from build123d import *

# Parameters (mm, degrees)
BOSS_EXTRUDE1_DEPTH = 3
SKETCH2_R           = 13.5
BOSS_EXTRUDE2_DEPTH = 5
SKETCH3_R           = 7.5
CUT_EXTRUDE1_DEPTH  = 1
SKETCH4_R           = 4
CUT_EXTRUDE2_DEPTH  = 9


with BuildPart() as part:
    # Sketch1 → Boss-Extrude1 (new body)
    with BuildSketch(Plane.XY):
        Polygon((5.773502692, -10), (11.547005384, 0), (5.773502692, 10), (-5.773502692, 10), (-11.547005384, 0), (-5.773502692, -10), align=None)
    extrude(amount=BOSS_EXTRUDE1_DEPTH)

    # Sketch2 → Boss-Extrude2 (add)
    with BuildSketch(Plane.XY.offset(3)):
        Circle(SKETCH2_R)
    extrude(amount=BOSS_EXTRUDE2_DEPTH)

    # Sketch3 → Cut-Extrude1 (cut)
    with BuildSketch(Plane.XY.offset(8)):
        Circle(SKETCH3_R)
    extrude(amount=-CUT_EXTRUDE1_DEPTH, mode=Mode.SUBTRACT)

    # Sketch4 → Cut-Extrude2 (cut, through all)
    with BuildSketch(Plane(origin=(0, 0, 0), x_dir=(-1, 0, 0), z_dir=(0, 0, -1))):
        Circle(SKETCH4_R)
    extrude(amount=-CUT_EXTRUDE2_DEPTH, mode=Mode.SUBTRACT)


solid = part.part
Verification items for the finished model (mm, model axes). A direction names the side the tool comes from. Give positions to 0.01 mm unless a question says otherwise; leave off trailing zeros. Loops run counter-clockwise (first coordinate to the right, second up) from the corner with the lowest first, then second, coordinate; pieces in that order, holes last. Notation, with made-up numbers: (85, 86) - (107, 86) arc R10 cw to (107, 103) - close; hole circle Ø7 at (38.25, 25.5). An arc over 180 degrees is marked (long way). Write item = value, one per line. Start each with the question number.
Q1. Cross-section at C-C, the plane y = 1. Enter the section's corners in (x, z).
Q2. Depth check by flat-ended pin: P1, Ø3, axis at x = 10, z = 2.5, coming from the -Y side; P2, Ø3, axis at y = -4.5, z = 6.5, coming from the +X side; P3, Ø1.5, axis at x = 9.5, z = 5.5, coming from the +Y side. Enter the tip coordinate at first touch or a pass-through.
Q3. Cross-section at A-A, the plane x = 3.5. Enter the section's corners in (y, z).
Q4. Thickness scan on line 1 (Y direction, x = 0, z = 7.4); line 2 (Y direction, x = 0, z = 2); line 3 (Z direction, x = 1.5, y = 4). Record the ranges inside material, lowest first.
Q5. Mould release check, pull along Y, two halves, no side actions. Record for faces 1 (the face through (0.867, -3.905, 3.451)), 2 (the face through (-8.7, -4.93, 1.48)), 3 (the face through (0, 10, 1)): released by +Y, released by -Y, zero draft, split by the parting line, or undercut.
Q6. Tool access check on faces 4 (the face through (8.62, -5.07, 1.48)), 5 (the face through (-8.62, 5.07, 1.48)), 6 (the face through (9, 5, 3)), 7 (the face through (-7.493, 0.33, 7.507)), 8 (the face through (8.7, 4.93, 1.48)). Record the directions out of +Z, -Z, +X, -X, +Y, -Y that give a thin tool (end or side, any length) a straight path to the whole face; none if there is none.
Q7. Cross-section at D-D, the plane z = 3.75. Enter the section's corners in (x, y).
Q8. Cross-section at B-B, the plane z = 1.25. Enter the section's corners in (x, y), and give its area (3 significant figures).
Answer key:
q1.outline = (-13.46, 3) - (-10.97, 3) - (-10.97, 0) - (-3.87, 0) - (-3.87, 7) - (-7.43, 7) - (-7.43, 8) - (-13.46, 8) - close; (3.87, 0) - (10.97, 0) - (10.97, 3) - (13.46, 3) - (13.46, 8) - (7.43, 8) - (7.43, 7) - (3.87, 7) - close
q2.P1 = -10.42
q2.P2 = 13.16
q2.P3 = 10.28
q3.outline = (-13.04, 3) - (-10, 3) - (-10, 0) - (-1.94, 0) - (-1.94, 7) - (-6.63, 7) - (-6.63, 8) - (-13.04, 8) - close; (1.94, 0) - (10, 0) - (10, 3) - (13.04, 3) - (13.04, 8) - (6.63, 8) - (6.63, 7) - (1.94, 7) - close
q4.line_1 = -13.5 to -7.5, 7.5 to 13.5
q4.line_2 = -10 to -4, 4 to 10
q4.line_3 = 0 to 7
q5.face_1 = undercut
q5.face_2 = released by -Y
q5.face_3 = released by +Y
q6.face_4 = -Z, +X, -Y
q6.face_5 = -Z, -X, +Y
q6.face_6 = -Z
q6.face_7 = +Z
q6.face_8 = -Z, +X, +Y
q7.outline = circle Ø27 at (0, 0); hole circle Ø8 at (0, 0)
q8.outline = (-11.55, 0) - (-5.77, -10) - (5.77, -10) - (11.55, 0) - (5.77, 10) - (-5.77, 10) - close; hole circle Ø8 at (0, 0)
q8.area = 296 mm^2
